from build123d import *

# Parameters (mm, degrees)
SKETCH1_W           = 30
SKETCH1_H           = 30
SKETCH1_W_2         = 26
SKETCH1_H_2         = 26
BOSS_EXTRUDE1_DEPTH = 2000
BOSS_EXTRUDE2_DEPTH = 10


with BuildPart() as part:
    # Sketch1 → Boss-Extrude1 (new body)
    with BuildSketch(Plane.XY):
        Rectangle(SKETCH1_W, SKETCH1_H)
        Rectangle(SKETCH1_W_2, SKETCH1_H_2, mode=Mode.SUBTRACT)
    extrude(amount=BOSS_EXTRUDE1_DEPTH)

    # Sketch2 → Boss-Extrude2 (add)
    with BuildSketch(Plane(origin=(15, 0, 0), x_dir=(0, 0, -1), z_dir=(1, 0, 0))):
        Polygon((-30, 15), (0, 15), (0, 45), (30, 45), (30, 15), (30, -15), (30, -45), (0, -45), (0, -15), (-30, -15), align=None)
    extrude(amount=BOSS_EXTRUDE2_DEPTH)


solid = part.part
CAD build for the part. Positions are in the model's coordinates, mm. Round coordinates to 2 decimals unless told otherwise and drop trailing zeros. Order: outer loops, then holes, each group sorted by start corner. A loop starts at its lowest first (then second) coordinate and runs counter-clockwise, first axis right, second up. Notation, with made-up numbers: M 52.5,78 L 95.5,78 A12 ccw 95.5,94 Z; hole C 22,19 d7. An arc over 180 degrees is marked long. Use one line per item in the form item = value.
Q1. Probe L1, parallel to Y at x = -9, z = 350; L2, parallel to X at y = 14.5, z = 1608.5. List the from-to ranges inside material, lowest first.
Recorded:
L1 = -15 to -13, 13 to 15
L2 = -15 to 15
Q2. Saw through at A-A on z = 291.5. Give the cut face in (x, y), then the cut area to 3 significant figures.
Recorded:
outline = M -15,-15 L 15,-15 L 15,15 L -15,15 Z; hole M -13,-13 L 13,-13 L 13,13 L -13,13 Z
area = 224 mm^2
Q3. Saw through at B-B on x = -3. Give the cut face in (y, z).
Recorded:
outline = M -15,0 L -13,0 L -13,2000 L -15,2000 Z; M 13,0 L 15,0 L 15,2000 L 13,2000 Z
Q4. Flat gauge pins, fed straight in: P1, Ø8, axis at x = 11, z = 735.5, coming from the +Y side; P2, Ø8, axis at x = 13, y = 33.5, coming from the +Z side; P3, Ø2, axis at x = 13, z = 1685, coming from the -Y side. Where does each tip first touch, or does it go through?
Recorded:
P1 = 15
P2 = 0
P3 = -15
